from build123d import *

# Parameters (mm, degrees)
SKETCH_1_W          = 25
SKETCH_1_H          = 30
EXTRUDE_1_DEPTH     = 60
SKETCH_2_R          = 9.6
CUT_EXTRUDE_1_DEPTH = 47.5
SKETCH_3_R          = 5.65
CUT_EXTRUDE_2_DEPTH = 13.5


with BuildPart() as part:
    # ｽｹｯﾁ1 → ﾎﾞｽ - 押し出し1 (new body)
    with BuildSketch(Plane.XY):
        with Locations((1.917887822, -3.131578947)):
            Rectangle(SKETCH_1_W, SKETCH_1_H)
    extrude(amount=EXTRUDE_1_DEPTH)

    # ｽｹｯﾁ2 → ｶｯﾄ - 押し出し1 (cut)
    with BuildSketch(Plane(origin=(0, 0, 0), x_dir=(-1, 0, 0), z_dir=(0, 0, -1))):
        with Locations((-1.917887822, -0.631578947)):
            Circle(SKETCH_2_R)
    extrude(amount=-CUT_EXTRUDE_1_DEPTH, mode=Mode.SUBTRACT)

    # ｽｹｯﾁ3 → ｶｯﾄ - 押し出し2 (cut, through all)
    with BuildSketch(Plane(origin=(0, 0, 47.5), x_dir=(-1, 0, 0), z_dir=(0, 0, -1))):
        with Locations((-1.917887822, -0.631578947)):
            Circle(SKETCH_3_R)
    extrude(amount=-CUT_EXTRUDE_2_DEPTH, mode=Mode.SUBTRACT)


solid = part.part
Design review of the part built by this model. Coordinates are the model's own, in mm. A direction names the side the tool comes from. Round coordinates to 2 decimals unless told otherwise and drop trailing zeros. Loops run counter-clockwise (first coordinate to the right, second up) from the corner with the lowest first, then second, coordinate; pieces in that order, holes last. Notation, with made-up numbers: (-8, 49.25) - (12, 49.25) arc R14 cw to (12, 71.25) - close; hole circle Ø10 at (57.25, 38.5). An arc over 180 degrees is marked (long way). One line per item, written item: value. Start each with the question number.
1) For faces 1 (the flat face through (-1, -6, 60)), 2 (the cylindrical face through (-7.24, 2.25, 23.42)), list the 3-axis set-ups (+Z, -Z, +X, -X, +Y, -Y) from which the entire face can be reached by the end or side of a thin tool; tool diameter is ignored.
2) Consider section A-A on y = 3. Give the boundary of the cut face in (x, z), then the cut area to 3 significant figures.
3) Draft analysis for pull direction Y (two halves, no side actions). For faces 3 (the flat face through (-2, -5, 47.5)), 4 (the flat face through (-10.582, -3, 30)), 5 (the flat face through (2, 11.868, 30)), state which applies: +Y half, -Y half, draft (parallel to the pull), parting line (faces both ways), or undercut.
4) To check wall thickness, follow L1, parallel to X at y = -8.5, z = 46; L2, parallel to Z at x = 9.5, y = -3; L3, parallel to X at y = 0.25, z = 4.5. State the ranges of each line that lie inside material, in increasing order. Write a range as from..to.
5) Consider section C-C on x = -6.5. Give the boundary of the cut face in (y, z).
6) Insertion check: pin 1 Ø5 at (x, y) = (-7.5, 3.5) entering from -Z; pin 2 Ø7 at (x, y) = (1.92, -0.63) entering from -Z. Each pin has a flat end and moves straight along its axis. Give the tip position at first contact, or say it passes through.
7) Consider section B-B on z = 12. Give the boundary of the cut face in (x, y).
8) Consider section D-D on y = -4.5. Give the boundary of the cut face in (x, z), then the cut area to 3 significant figures.
Reported:
1. face 1: +Z, +X, -X, +Y, -Y
1. face 2: -Z
2. outline: (-10.58, 0) - (-6.97, 0) - (-6.97, 47.5) - (-2.41, 47.5) - (-2.41, 60) - (-10.58, 60) - close; (6.25, 47.5) - (10.8, 47.5) - (10.8, 0) - (14.42, 0) - (14.42, 60) - (6.25, 60) - close
2. area: 548 mm^2
3. face 3: undercut
3. face 4: draft
3. face 5: +Y half
4. L1: x = -10.58..-3.58, 7.42..14.42
4. L2: z = 47.5..60
4. L3: x = -10.58..-7.64, 11.48..14.42
5. outline: (-18.13, 0) - (-5.25, 0) - (-5.25, 47.5) - (3.98, 47.5) - (3.98, 0) - (11.87, 0) - (11.87, 60) - (-18.13, 60) - close
6. pin 1: stops at z = 0
6. pin 2: passes through
7. outline: (-10.58, -18.13) - (14.42, -18.13) - (14.42, 11.87) - (-10.58, 11.87) - close; hole circle Ø19.2 at (1.92, -0.63)
8. outline: (-10.58, 0) - (-6.87, 0) - (-6.87, 47.5) - (-2.2, 47.5) - (-2.2, 60) - (-10.58, 60) - close; (6.04, 47.5) - (10.7, 47.5) - (10.7, 0) - (14.42, 0) - (14.42, 60) - (6.04, 60) - close
8. area: 562 mm^2
